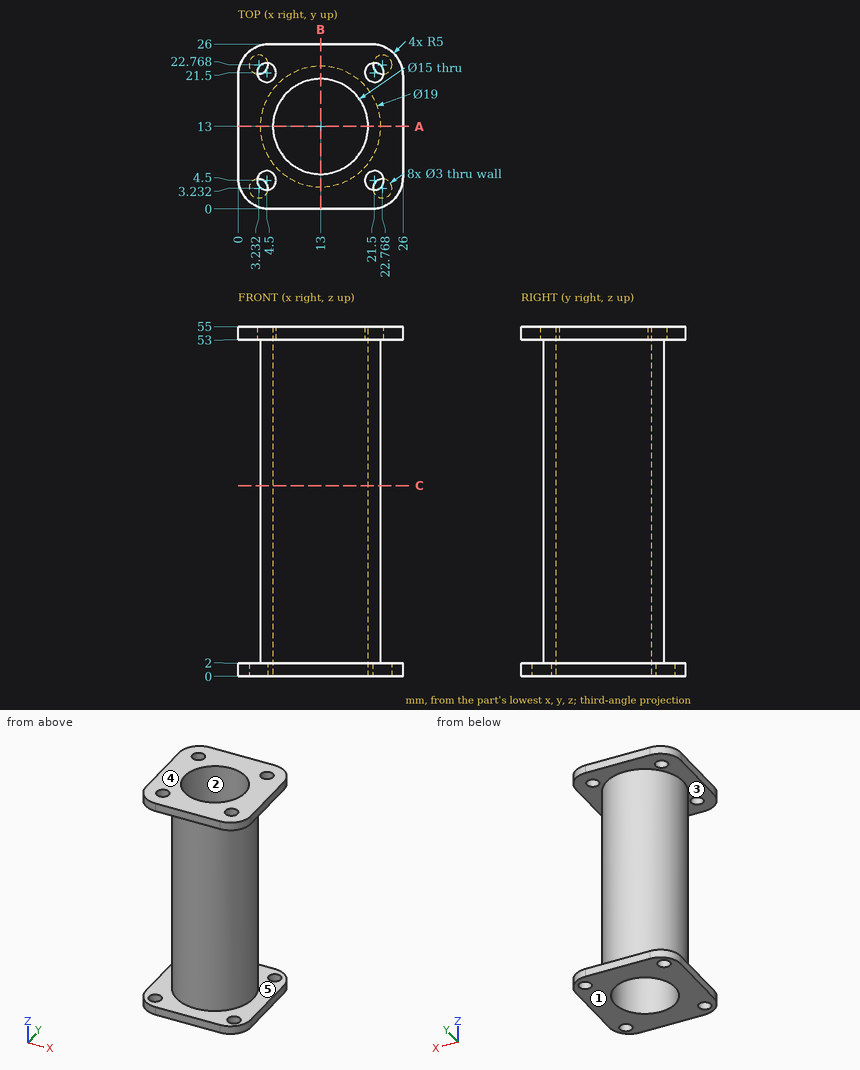
Design review of the part shown in the three views and the two pictorial views. Dimensions are in mm from the part's minimum x, y and z. A direction names the side the tool comes from. Give positions to 0.01 mm unless a question says otherwise; leave off trailing zeros. Write each loop counter-clockwise with the first axis right and the second up, starting at its lowest first coordinate (ties: lowest second). Pieces come first, ordered by that corner, then holes. Notation, with made-up numbers: M 23.25,-12.75 L 50.25,-12.75 A19 ccw 50.25,5.25 Z; hole C 85,28 d2. An arc over 180 degrees is marked long. Return JSON: item names as keys, results as strings. Group by question number.
Item 1: Clearance check with flat-ended pins moving along their axes: pin 1 Ø1 at (x, z) = (10, 14.5) entering from -Y (1 decimal); pin 2 Ø1 at (x, z) = (11.5, 6.5) entering from -Y; pin 3 Ø2.5 at (x, y) = (3.23, 3.23) entering from -Z. State where each tip first meets the part, or that it passes through.
Item 2: Tool access review of the marked faces 4 and 5: name each direction out of +Z, -Z, +X, -X, +Y, -Y from which nothing blocks a thin tool from reaching the whole face with its end or side.
Item 3: Take a section at C-C (z = 30). Give the boundary of the cut face in (x, y).
Item 4: The part is to be moulded in two halves that separate along Z. For the marked faces 1, 2 and 3, say which applies: pulls with the +Z half, pulls with the -Z half, needs draft (parallel to the pull), parting line crosses it, or undercut.
Item 5: Take a section at A-A (y = 13). Give the boundary of the cut face in (x, z), plus the area to 3 significant figures.
Item 6: Wall thickness on line 1 along Z through (x, y) = (2.5, 7.5); line 2 along Y through (x, z) = (4.5, 54.45) (1 decimal); line 3 along X through (y, z) = (19, 15) (1 decimal): over which ranges is each line inside the solid? List them lowest first.
Return value:
{
 "1": {"pin 1": "stops at y = 3.8", "pin 2": "stops at y = 3.55", "pin 3": "stops at z = 53"},
 "2": {"face 4": "+Z, +X, -X, +Y, -Y", "face 5": "none"},
 "3": {"outline": "C 13,13 d19; hole C 13,13 d15"},
 "4": {"face 1": "pulls with the -Z half", "face 2": "needs draft", "face 3": "undercut"},
 "5": {"outline": "M 0,0 L 5.5,0 L 5.5,55 L 0,55 L 0,53 L 3.5,53 L 3.5,2 L 0,2 Z; M 20.5,0 L 26,0 L 26,2 L 22.5,2 L 22.5,53 L 26,53 L 26,55 L 20.5,55 Z", "area": "248 mm2"},
 "6": {"line 1": "z = 0 to 2, 53 to 55", "line 2": "y = 0 to 3, 6 to 20, 23 to 26", "line 3": "x = 5.6 to 8.5, 17.5 to 20.4"}
}
